Source: CAD feature listing. Evaluate the final solid. Frame: model axes, mm. A direction names the side the tool comes from. Give positions to 0.01 mm unless a question says otherwise; leave off trailing zeros. Loops run counter-clockwise (first coordinate to the right, second up) from the corner with the lowest first, then second, coordinate; pieces in that order, holes last. Notation, with made-up numbers: M 75.5,54.25 L 112.5,54.25 A14 ccw 112.5,62.25 Z; hole C 70,-5.75 d4. An arc over 180 degrees is marked long. Answer in a Markdown table with one row per item.
```python
from build123d import *


with BuildPart() as part:
    # Sketch1 → Revolve1 (revolve)
    with BuildSketch(Plane.XY, mode=Mode.PRIVATE) as revolve1_sk:
        with BuildLine():
            Line((-35, 35), (-35, 25))
            Line((-35, 25), (-46.913025467, 5.144957554))
            ThreePointArc((-46.913025467, 5.144957554), (-48.33809621, 0), (-46.913025467, -5.144957554))
            Line((-46.913025467, -5.144957554), (-35, -25))
            Line((-35, -25), (-35, -35))
            Line((-35, -35), (-36.5, -35))
            Line((-36.5, -35), (-36.5, -25.415475947))
            Line((-36.5, -25.415475947), (-48.662311036, -5.144957554))
            ThreePointArc((-48.662311036, -5.144957554), (-50.087381779, 0), (-48.662311036, 5.144957554))
            Line((-48.662311036, 5.144957554), (-36.5, 25.415475947))
            Line((-36.5, 25.415475947), (-36.5, 35))
            Line((-36.5, 35), (-35, 35))
        make_face()
    revolve(revolve1_sk.sketch.rotate(Axis((0, 85.826086957, 0), (0, -1, 0)), 270), axis=Axis((0, 85.826086957, 0), (0, -1, 0)))


solid = part.part
```
Q1. Section query D-D (y = 9). Output: boundary loops of the cut face in (x, z).
Values follow:
| item | result |
|---|---|
| outline | C 0,0 d92.7; hole C 0,0 d89.2 |
Q2. Reachability of faces 4 (the cylindrical face through (21, 30, -28)), 5 (the cylindrical face through (35.632, 30.275, -7.912)), 6 (the conical face through (21.65, -24.04, -28.23)) from +Z, -Z, +X, -X, +Y, -Y: full face, straight path, thin tool, end or side. Return the list, or none.
Values follow:
| item | result |
|---|---|
| face 4 | +Y, -Y |
| face 5 | +Y |
| face 6 | none |
Q3. Contact query for flat-ended pins moving along their axis: pin 1 Ø1.5 at (y, z) = (19, -36.5) entering from +X; pin 2 Ø1 at (x, z) = (-36.5, -30.5) entering from -Y; pin 3 Ø5 at (x, y) = (14.5, 10) entering from +Z. Output: stop coordinate, or through.
Values follow:
| item | result |
|---|---|
| pin 1 | x = 19 |
| pin 2 | y = -7.81 |
| pin 3 | z = 45.15 |
Q4. Ray query, probe 1 along X at (y, z) = (29.25, 0); probe 2 along Y at (x, z) = (19.5, 32); probe 3 along Z at (x, y) = (21, -32). Return the intervals inside material, ascending. Write a range as from..to.
Values follow:
| item | result |
|---|---|
| probe 1 | -36.5..-35, 35..36.5 |
| probe 2 | -23.79..-20.88, 20.88..23.79 |
| probe 3 | -29.85..-28, 28..29.85 |
Q5. Section query A-A (x = 0). Output: boundary loops of the cut face in (y, z).
Values follow:
| item | result |
|---|---|
| outline | M -35,-36.5 L -25.42,-36.5 L -5.14,-48.66 A10 ccw 5.14,-48.66 L 25.42,-36.5 L 35,-36.5 L 35,-35 L 25,-35 L 5.14,-46.91 A10 cw -5.14,-46.91 L -25,-35 L -35,-35 Z; M -35,35 L -25,35 L -5.14,46.91 A10 cw 5.14,46.91 L 25,35 L 35,35 L 35,36.5 L 25.42,36.5 L 5.14,48.66 A10 ccw -5.14,48.66 L -25.42,36.5 L -35,36.5 Z |
Q6. Mould query, pull axis X, two halves, no side actions, for faces 1 (the cylindrical face through (35.632, -30.141, -7.912)), 2 (the flat face through (30, 35, 19)), 3 (the conical face through (-10.74, 23.76, 34.09)). Classes: +X half, -X half, draft (parallel to the pull), parting line (faces both ways), or undercut.
Values follow:
| item | result |
|---|---|
| face 1 | parting line |
| face 2 | draft |
| face 3 | undercut |
Q7. Section query B-B (z = 0). Output: boundary loops of the cut face in (x, y).
Values follow:
| item | result |
|---|---|
| outline | M -48.66,-5.14 L -36.5,-25.42 L -36.5,-35 L -35,-35 L -35,-25 L -46.91,-5.14 A10 cw -46.91,5.14 L -35,25 L -35,35 L -36.5,35 L -36.5,25.42 L -48.66,5.14 A10 ccw Z; M 35,-35 L 36.5,-35 L 36.5,-25.42 L 48.66,-5.14 A10 ccw 48.66,5.14 L 36.5,25.42 L 36.5,35 L 35,35 L 35,25 L 46.91,5.14 A10 cw 46.91,-5.14 L 35,-25 Z |
Q8. Section query C-C (y = 30). Output: boundary loops of the cut face in (x, z).
Values follow:
| item | result |
|---|---|
| outline | C 0,0 d73; hole C 0,0 d70 |
